Here's how the part is built. I have some questions about the finished solid (model axes, mm). Round coordinates to 2 decimals unless told otherwise and drop trailing zeros. Write each loop counter-clockwise with the first axis right and the second up, starting at its lowest first coordinate (ties: lowest second). Pieces come first, ordered by that corner, then holes. Notation, with made-up numbers: (70.5, -14.75) - (102.5, -14.75) arc R24 cw to (102.5, 2.25) - close; hole circle Ø3 at (38, -11.75). An arc over 180 degrees is marked (long way). One line per question, with ' | ' between items. Start each with the question number.
(1) Imagine slicing it at A-A (y = -37). Write out the boundary of the cut face in (x, z).
(2) If I drill on L1, parallel to Z at x = 6.5, y = 288.5; L2, parallel to X at y = 63, z = 1.5, over which ranges is the centre line in solid material (lowest first)?
(3) Will these pins go through, and if not, where does the flat tip stop? pin 1 (1 mm diameter, centred on x = 0.5, y = -94, fed in from +Z); pin 2 (2.5 mm diameter, centred on y = 136, z = 1, fed in from +X); pin 3 (2.5 mm diameter, centred on x = 0, y = 69.5, fed in from -Z).
from build123d import *

# Parameters (mm, degrees)
BOSS_EXTRUDE1_DEPTH      = 368.3
BOSS_EXTRUDE1_DEPTH_BACK = 368.3
SKETCH1_W                = 20
SKETCH1_H                = 20
CUT_EXTRUDE1_DEPTH       = 369.571417774
CUT_EXTRUDE1_DEPTH_BACK  = 369.571417774
SKETCH2_W                = 5
SKETCH2_H                = 12
SKETCH2_W_2              = 12
SKETCH2_H_2              = 5


with BuildPart() as part:
    # Sketch1 → Boss-Extrude1 (new, two sides: drawn at the far end of the back side and taken through both)
    with BuildSketch(Plane(origin=(0, 0, 0), x_dir=(1, 0, 0), z_dir=(0, 1, 0)).offset(-BOSS_EXTRUDE1_DEPTH_BACK)):
        Rectangle(SKETCH1_W, SKETCH1_H)
    extrude(amount=BOSS_EXTRUDE1_DEPTH + BOSS_EXTRUDE1_DEPTH_BACK)

    # Sketch2 → Cut-Extrude1 (cut, two sides: drawn at the far end of the back side and taken through both)
    with BuildSketch(Plane(origin=(0, 0, 0), x_dir=(1, 0, 0), z_dir=(0, 1, 0)).offset(-CUT_EXTRUDE1_DEPTH_BACK)):
        with Locations((0, 10)):
            Rectangle(SKETCH2_W, SKETCH2_H)
        with Locations((10, 0)):
            Rectangle(SKETCH2_W_2, SKETCH2_H_2)
        with Locations((-10, 0)):
            Rectangle(SKETCH2_W_2, SKETCH2_H_2)
        with Locations((0, -10)):
            Rectangle(SKETCH2_W, SKETCH2_H)
    extrude(amount=CUT_EXTRUDE1_DEPTH + CUT_EXTRUDE1_DEPTH_BACK, mode=Mode.SUBTRACT)


solid = part.part
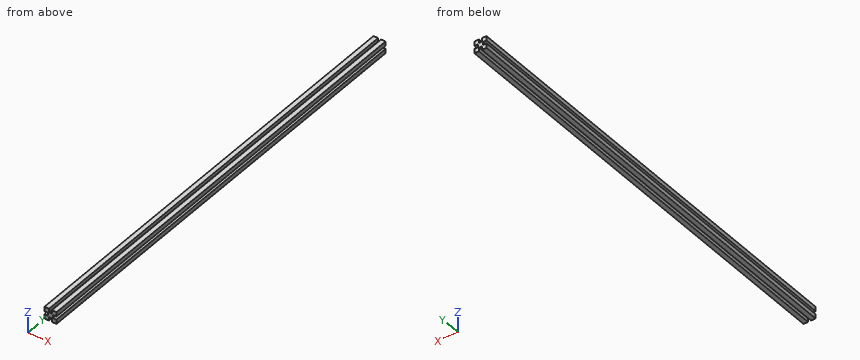
Check sheet entries:
1) outline: (-10, -10) - (-2.5, -10) - (-2.5, -4) - (2.5, -4) - (2.5, -10) - (10, -10) - (10, -2.5) - (4, -2.5) - (4, 2.5) - (10, 2.5) - (10, 10) - (2.5, 10) - (2.5, 4) - (-2.5, 4) - (-2.5, 10) - (-10, 10) - (-10, 2.5) - (-4, 2.5) - (-4, -2.5) - (-10, -2.5) - close
2) L1: -10 to -2.5, 2.5 to 10 | L2: -4 to 4
3) pin 1: z = 4 | pin 2: x = 4 | pin 3: z = -4
